Here's how the part is built. I have some questions about the finished solid (model axes, mm). A direction names the side the tool comes from. Round coordinates to 2 decimals unless told otherwise and drop trailing zeros. Order: outer loops, then holes, each group sorted by start corner. A loop starts at its lowest first (then second) coordinate and runs counter-clockwise, first axis right, second up.
```python
from build123d import *

# Parameters (mm, degrees)
BOSS_EXTRUDE1_DEPTH = 17.5
SKETCH2_W           = 18
SKETCH2_H           = 5
CUT_EXTRUDE1_DEPTH  = 17.5
SKETCH3_R           = 1.625
CUT_EXTRUDE2_DEPTH  = 5
SKETCH4_R           = 3
CUT_EXTRUDE3_DEPTH  = 2
CHAMFER1_SIZE       = 2
SKETCH5_W           = 12.7
SKETCH5_H           = 6.35
CUT_EXTRUDE4_DEPTH  = 5


with BuildPart() as part:
    # Sketch1 → Boss-Extrude1 (new, symmetric)
    with BuildSketch(Plane.XY):
        with BuildLine():
            Line((-75, 17.5), (75, 17.5))
            ThreePointArc((75, 17.5), (81.614378278, 16.201851746), (87.247448714, 12.5))
            Line((87.247448714, 12.5), (-87.247448714, 12.5))
            ThreePointArc((-87.247448714, 12.5), (-81.614378278, 16.201851746), (-75, 17.5))
        make_face()
    extrude(amount=BOSS_EXTRUDE1_DEPTH, both=True)

    # Sketch2 → Cut-Extrude1 (cut, symmetric)
    with BuildSketch(Plane.XY):
        with Locations((-78.247448714, 15)):
            Rectangle(SKETCH2_W, SKETCH2_H)
    extrude(amount=CUT_EXTRUDE1_DEPTH, both=True, mode=Mode.SUBTRACT)

    # Sketch3 → Cut-Extrude2 (cut)
    with BuildSketch(Plane.XZ.offset(-12.5)):
        with Locations((-46, -10)):
            Circle(SKETCH3_R)
        with Locations((-9.833333333, -10)):
            Circle(SKETCH3_R)
        with Locations((26.333333333, -10)):
            Circle(SKETCH3_R)
        with Locations((62.5, -10)):
            Circle(SKETCH3_R)
    cut_extrude2 = extrude(amount=-CUT_EXTRUDE2_DEPTH, mode=Mode.SUBTRACT)

    # Sketch4 → Cut-Extrude3 (cut)
    with BuildSketch(Plane(origin=(0, 17.5, 0), x_dir=(1, 0, 0), z_dir=(0, 1, 0))):
        with Locations(Location((62.5, 9.9, 0), (0, 0, 180))):
            Circle(SKETCH4_R)
        with Locations(Location((26.333333333, 9.9, 0), (0, 0, 180))):
            Circle(SKETCH4_R)
        with Locations(Location((-9.833333333, 10, 0), (0, 0, 180))):
            Circle(SKETCH4_R)
        with Locations(Location((-46, 10, 0), (0, 0, 180))):
            Circle(SKETCH4_R)
    cut_extrude3 = extrude(amount=-CUT_EXTRUDE3_DEPTH, mode=Mode.SUBTRACT)

    # Mirror1: Cut-Extrude2, Cut-Extrude3 across plane
    add(cut_extrude2.mirror(Plane.XY), mode=Mode.SUBTRACT)
    add(cut_extrude3.mirror(Plane.XY), mode=Mode.SUBTRACT)

    # Chamfer1
    chamfer1_edges = [part.edges().sort_by_distance(p)[0] for p in [
        (81.614378278, 16.201851746, 17.5),
        (2.876275643, 17.5, 17.5),
        (2.876275643, 17.5, -17.5),
        (81.614378278, 16.201851746, -17.5),
    ]]
    chamfer(chamfer1_edges, length=CHAMFER1_SIZE)

    # Sketch5 → Cut-Extrude4 (cut)
    with BuildSketch(Plane(origin=(0, 17.5, 0), x_dir=(1, 0, 0), z_dir=(0, 1, 0))):
        with Locations((-62.897448714, -8.5)):
            Rectangle(SKETCH5_W, SKETCH5_H)
    extrude(amount=-CUT_EXTRUDE4_DEPTH, mode=Mode.SUBTRACT)


solid = part.part
```
1) We'd pull the mould along X, two halves only. Please class faces 4 (the cylindrical face through (64.05, 13.98, 9.51)), 5 (the conical face through (81.065, 15.09, -16.736)), 6 (the flat face through (-63, 15, 11.675)), 7 (the flat face through (-56.547, 15, 9)): +X half, -X half, draft (parallel to the pull), parting line (faces both ways), or undercut.
2) If we section it at C-C (y = 13.55): Give the number of separate pieces and of enclosed holes in the cut face, plus the area to 3 significant figures.
3) I'm going to push flat-ended pins straight in: pin 1 (1.8 mm diameter, centred on x = 61.5, z = 8.5, fed in from +Y); pin 2 (1.9 mm diameter, centred on x = -9.83, z = 10, fed in from -Y). Where does each tip first touch, or does it pass through?
4) If we section it at A-A (x = -54.5): Write out the boundary of the cut face in (y, z), plus the area to 3 significant figures.
5) For faces 1 (the flat face through (61, 15.5, -11)), 2 (the cylindrical face through (24.71, 13.98, 9.93)), 3 (the flat face through (-63, 15, 5.325)), which set-ups out of +Z, -Z, +X, -X, +Y, -Y let a thin tool reach every point of the face, with its end or its side?
6) I need wall thicknesses on line 1 (Z direction, x = 62.5, y = 13.1) (3 decimals); line 2 (X direction, y = 13.4, z = 11); line 3 (X direction, y = 13.95, z = 10) (3 decimals). Which ranges of each line are inside material? Lowest first, please.
7) If we section it at B-B (z = -5): Write out the boundary of the cut face in (x, y).
Solutions:
1. face 4: undercut
1. face 5: +X half
1. face 6: draft
1. face 7: -X half
2. separate pieces: 1
2. enclosed holes: 8
2. area: 5,280 mm2
3. pin 1: stops at y = 15.5
3. pin 2: passes through
4. outline: (12.5, -17.5) - (15.5, -17.5) - (17.5, -15.5) - (17.5, 15.5) - (15.5, 17.5) - (12.5, 17.5) - close
4. area: 171 mm2
5. face 1: +Y
5. face 2: +Y, -Y
5. face 3: -X, +Y, -Y
6. line 1: z = -17.5 to -11.625, -8.375 to 8.375, 11.625 to 17.5
6. line 2: x = -56.55 to -47.28, -44.72 to -11.11, -8.55 to 25.05, 27.61 to 61.22, 63.78 to 86.26
6. line 3: x = -56.547 to -47.625, -44.375 to -11.458, -8.208 to 24.708, 27.958 to 60.875, 64.125 to 85.566
7. outline: (-69.25, 12.5) - (87.25, 12.5) arc R17.5 ccw to (75, 17.5) - (-69.25, 17.5) - close
